Design review of the part built by this model. Coordinates are the model's own, in mm. Coordinates: 2 decimals unless noted, no trailing zeros. Loops run counter-clockwise (first coordinate to the right, second up) from the corner with the lowest first, then second, coordinate; pieces in that order, holes last.
from build123d import *

# Parameters (mm, degrees)
BOSS_EXTRUDE1_DEPTH = 101.6
SKETCH3_R           = 2.54
CUT_EXTRUDE1_DEPTH  = 4.175
SKETCH4_R           = 2.54
CUT_EXTRUDE2_DEPTH  = 4.175


with BuildPart() as part:
    # Sketch2 → Boss-Extrude1 (new body)
    with BuildSketch(Plane(origin=(0, 0, 0), x_dir=(1, 0, 0), z_dir=(0, 1, 0))):
        Polygon((-25.4, 25.4), (-25.4, -25.4), (-22.225, -25.4), (-22.225, 22.225), (25.4, 22.225), (25.4, 25.4), align=None)
    extrude(amount=BOSS_EXTRUDE1_DEPTH)

    # Sketch3 → Cut-Extrude1 (cut, through all)
    with BuildSketch(Plane.XY.offset(-22.225)):
        with Locations((12.7, 88.9)):
            Circle(SKETCH3_R)
        with Locations((0, 88.9)):
            Circle(SKETCH3_R)
        with Locations((0, 63.5)):
            Circle(SKETCH3_R)
        with Locations((12.7, 63.5)):
            Circle(SKETCH3_R)
        with Locations((0, 38.1)):
            Circle(SKETCH3_R)
        with Locations((12.7, 38.1)):
            Circle(SKETCH3_R)
        with Locations((0, 12.7)):
            Circle(SKETCH3_R)
        with Locations((12.7, 12.7)):
            Circle(SKETCH3_R)
    extrude(amount=-CUT_EXTRUDE1_DEPTH, mode=Mode.SUBTRACT)

    # Sketch4 → Cut-Extrude2 (cut, through all)
    with BuildSketch(Plane(origin=(-22.225, 0, 0), x_dir=(0, 0, -1), z_dir=(1, 0, 0))):
        with Locations((-12.7, 88.9)):
            Circle(SKETCH4_R)
        with Locations((0, 88.9)):
            Circle(SKETCH4_R)
        with Locations((-12.7, 63.5)):
            Circle(SKETCH4_R)
        with Locations((0, 63.5)):
            Circle(SKETCH4_R)
        with Locations((-12.7, 38.1)):
            Circle(SKETCH4_R)
        with Locations((0, 38.1)):
            Circle(SKETCH4_R)
        with Locations((-12.7, 12.7)):
            Circle(SKETCH4_R)
        with Locations((0, 12.7)):
            Circle(SKETCH4_R)
    extrude(amount=-CUT_EXTRUDE2_DEPTH, mode=Mode.SUBTRACT)


solid = part.part
Q1. For line 1 (Y direction, x = -24.5, z = 0); line 2 (X direction, y = 24.5, z = -11) (3 decimals), list the stretches that pass through material, from the lowest coordinate up.
Q2. Clearance check with flat-ended pins moving along their axes: pin 1 Ø3 at (y, z) = (12.7, 0) entering from -X; pin 2 Ø6.5 at (x, y) = (0, 12.7) entering from +Z (3 decimals); pin 3 Ø6 at (y, z) = (38.1, 0) entering from +X (3 decimals). State where each tip first meets the part, or that it passes through.
Q3. Take a section at C-C, the plane z = 0. Write out the cut boundary in (x, y) (3 decimals).
Q4. The part is to be moulded in two halves that separate along Z. For faces 1 (the cylindrical face through (-23.79, 87.354, 14.716)), 2 (the flat face through (1, 50, -22.225)), 3 (the cylindrical face through (12.15, 61.02, -23.79)), 4 (the cylindrical face through (-23.79, 61.02, 0.55)), say which applies: pulls with the +Z half, pulls with the -Z half, needs draft (parallel to the pull), parting line crosses it, or undercut.
Q5. Take a section at A-A, the plane y = 12.7. Write out the cut boundary in (x, z) (3 decimals).
Q6. Take a section at D-D, the plane y = 62.5. Write out the cut boundary in (x, z) (3 decimals).
Q7. Take a section at B-B, the plane x = 0. Write out the cut boundary in (y, z) (3 decimals), then the cut area to 3 significant figures.
Entries:
1. line 1: y = 0 to 10.16, 15.24 to 35.56, 40.64 to 60.96, 66.04 to 86.36, 91.44 to 101.6
1. line 2: x = -25.4 to -22.225
2. pin 1: passes through
2. pin 2: stops at z = -22.225
2. pin 3: stops at x = -22.225
3. outline: (-25.4, 0) - (-22.225, 0) - (-22.225, 10.16) - (-25.4, 10.16) - close; (-25.4, 15.24) - (-22.225, 15.24) - (-22.225, 35.56) - (-25.4, 35.56) - close; (-25.4, 40.64) - (-22.225, 40.64) - (-22.225, 60.96) - (-25.4, 60.96) - close; (-25.4, 66.04) - (-22.225, 66.04) - (-22.225, 86.36) - (-25.4, 86.36) - close; (-25.4, 91.44) - (-22.225, 91.44) - (-22.225, 101.6) - (-25.4, 101.6) - close
4. face 1: undercut
4. face 2: pulls with the +Z half
4. face 3: needs draft
4. face 4: undercut
5. outline: (-25.4, -25.4) - (-2.54, -25.4) - (-2.54, -22.225) - (-22.225, -22.225) - (-22.225, -2.54) - (-25.4, -2.54) - close; (-25.4, 2.54) - (-22.225, 2.54) - (-22.225, 10.16) - (-25.4, 10.16) - close; (-25.4, 15.24) - (-22.225, 15.24) - (-22.225, 25.4) - (-25.4, 25.4) - close; (2.54, -25.4) - (10.16, -25.4) - (10.16, -22.225) - (2.54, -22.225) - close; (15.24, -25.4) - (25.4, -25.4) - (25.4, -22.225) - (15.24, -22.225) - close
6. outline: (-25.4, -25.4) - (-2.335, -25.4) - (-2.335, -22.225) - (-22.225, -22.225) - (-22.225, -2.335) - (-25.4, -2.335) - close; (-25.4, 2.335) - (-22.225, 2.335) - (-22.225, 10.365) - (-25.4, 10.365) - close; (-25.4, 15.035) - (-22.225, 15.035) - (-22.225, 25.4) - (-25.4, 25.4) - close; (2.335, -25.4) - (10.365, -25.4) - (10.365, -22.225) - (2.335, -22.225) - close; (15.035, -25.4) - (25.4, -25.4) - (25.4, -22.225) - (15.035, -22.225) - close
7. outline: (0, -25.4) - (10.16, -25.4) - (10.16, -22.225) - (0, -22.225) - close; (15.24, -25.4) - (35.56, -25.4) - (35.56, -22.225) - (15.24, -22.225) - close; (40.64, -25.4) - (60.96, -25.4) - (60.96, -22.225) - (40.64, -22.225) - close; (66.04, -25.4) - (86.36, -25.4) - (86.36, -22.225) - (66.04, -22.225) - close; (91.44, -25.4) - (101.6, -25.4) - (101.6, -22.225) - (91.44, -22.225) - close
7. area: 258 mm2
